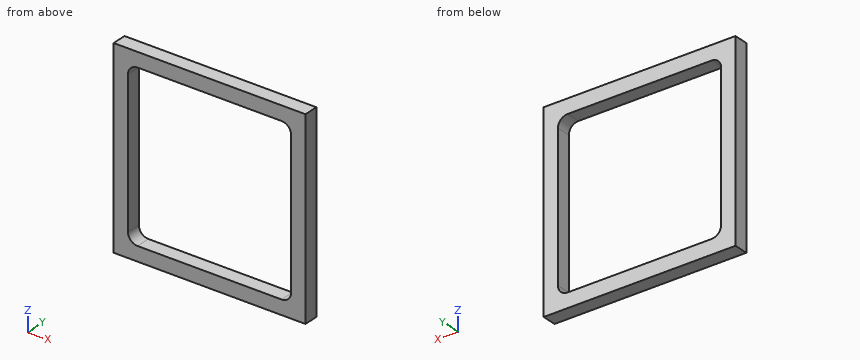
from build123d import *

# Parameters (mm, degrees)
SKETCH1_W           = 127.635
SKETCH1_H           = 127.635
BOSS_EXTRUDE1_DEPTH = 9.525
SKETCH5_W           = 108.585
SKETCH5_H           = 108.585
CUT_EXTRUDE1_DEPTH  = 9.525
FILLET1_R           = 6.35


with BuildPart() as part:
    # Sketch1 → Boss-Extrude1 (new body)
    with BuildSketch(Plane(origin=(0, 0, 0), x_dir=(1, 0, 0), z_dir=(0, 1, 0))):
        with Locations((63.8175, 63.8175)):
            Rectangle(SKETCH1_W, SKETCH1_H)
    extrude(amount=BOSS_EXTRUDE1_DEPTH)

    # Sketch5 → Cut-Extrude1 (cut)
    with BuildSketch(Plane(origin=(0, 9.525, 0), x_dir=(1, 0, 0), z_dir=(0, 1, 0))):
        with Locations((63.8175, 63.8175)):
            Rectangle(SKETCH5_W, SKETCH5_H)
    extrude(amount=-CUT_EXTRUDE1_DEPTH, mode=Mode.SUBTRACT)

    # Fillet1
    fillet1_edges = [part.edges().sort_by_distance(p)[0] for p in [
        (118.11, 4.7625, -9.525),
        (9.525, 4.7625, -9.525),
        (9.525, 4.7625, -118.11),
        (118.11, 4.7625, -118.11),
    ]]
    fillet(fillet1_edges, radius=FILLET1_R)


solid = part.part
Verification items for the finished model (mm, model axes). Coordinates: 2 decimals unless noted, no trailing zeros. Loops run counter-clockwise (first coordinate to the right, second up) from the corner with the lowest first, then second, coordinate; pieces in that order, holes last. Notation, with made-up numbers: (39.25, -34) -> (80.25, -34) arc R5 cw to (80.25, -30) -> close; hole circle Ø5 at (18, 68). An arc over 180 degrees is marked (long way). Answer as CSV lines item,"result".
1) Cross-section at C-C, the plane z = -39. Record the cut outline in (x, y) (3 decimals).
Found:
outline,"(0, 0) -> (9.525, 0) -> (9.525, 9.525) -> (0, 9.525) -> close; (118.11, 0) -> (127.635, 0) -> (127.635, 9.525) -> (118.11, 9.525) -> close"
2) Thickness scan on L1, parallel to Z at x = 94.5, y = 4 (3 decimals); L2, parallel to X at y = 5.75, z = -65 (3 decimals); L3, parallel to X at y = 3.5, z = -117 (3 decimals). Record the ranges inside material, lowest first. Write a range as from..to.
Found:
L1,"z = -127.635..-118.11, -9.525..0"
L2,"x = 0..9.525, 118.11..127.635"
L3,"x = 0..12.288, 115.347..127.635"
3) Cross-section at A-A, the plane x = 30.5. Record the cut outline in (y, z) (3 decimals).
Found:
outline,"(0, -127.635) -> (9.525, -127.635) -> (9.525, -118.11) -> (0, -118.11) -> close; (0, -9.525) -> (9.525, -9.525) -> (9.525, 0) -> (0, 0) -> close"
4) Cross-section at B-B, the plane y = 6.25. Record the cut outline in (x, z) (3 decimals), then the cut area to 3 significant figures.
Found:
outline,"(0, -127.635) -> (127.635, -127.635) -> (127.635, 0) -> (0, 0) -> close; hole (9.525, -111.76) arc R6.35 ccw to (15.875, -118.11) -> (111.76, -118.11) arc R6.35 ccw to (118.11, -111.76) -> (118.11, -15.875) arc R6.35 ccw to (111.76, -9.525) -> (15.875, -9.525) arc R6.35 ccw to (9.525, -15.875) -> close"
area,"4,530 mm2"
